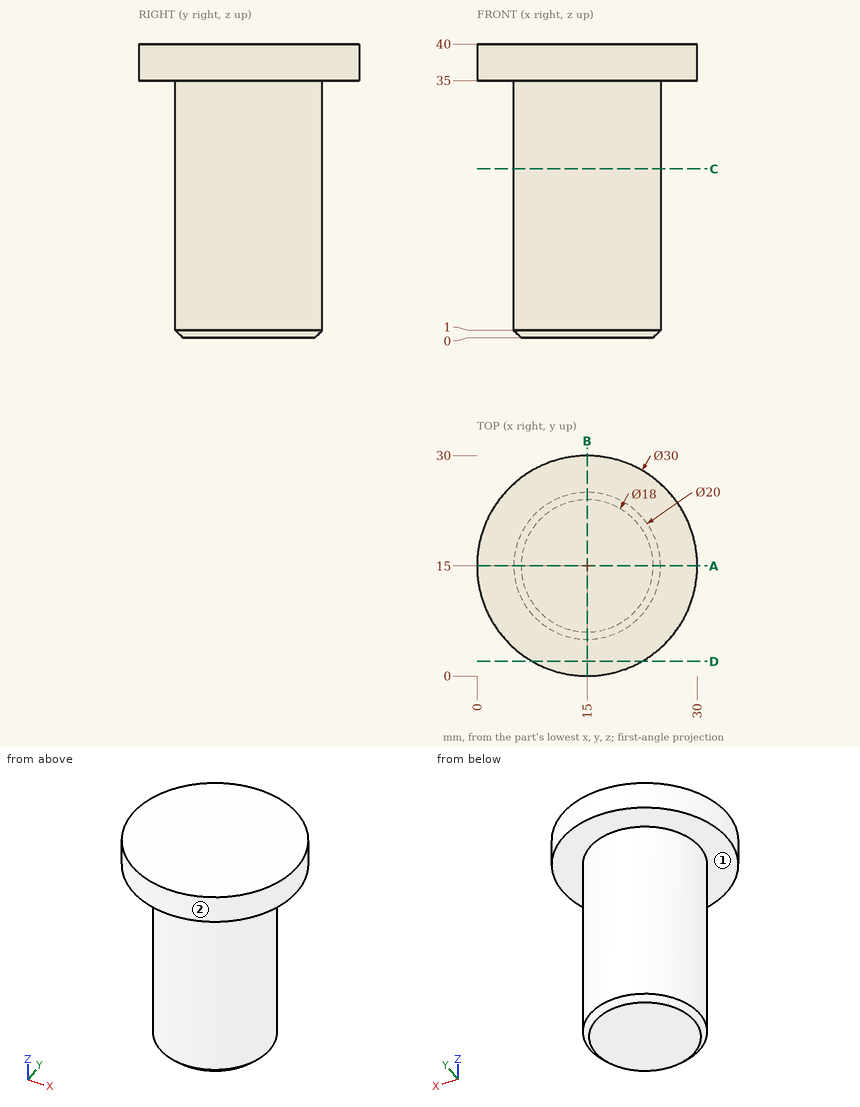
Design review of the part shown in the three views and the two pictorial views. Dimensions are in mm from the part's minimum x, y and z. A direction names the side the tool comes from. Coordinates: 2 decimals unless noted, no trailing zeros. Loops run counter-clockwise (first coordinate to the right, second up) from the corner with the lowest first, then second, coordinate; pieces in that order, holes last. Notation, with made-up numbers: (22.25, 83) - (59.25, 83) arc R10 ccw to (59.25, 88) - close; hole circle Ø11 at (82, 39.5). An arc over 180 degrees is marked (long way). Use a Markdown table: item, result. Add a question column.
Item 1: Tool access review of the marked faces 1 and 2: name each direction out of +Z, -Z, +X, -X, +Y, -Y from which nothing blocks a thin tool from reaching the whole face with its end or side.
Item 2: Insertion check: pin 1 Ø4 at (y, z) = (13, 4.5) entering from -X; pin 2 Ø5 at (y, z) = (17.5, 8.5) entering from +X; pin 3 Ø1 at (y, z) = (5.5, 30) entering from -X; pin 4 Ø1.5 at (x, y) = (11.5, 11.5) entering from -Z. Each pin has a flat end and moves straight along its axis. Give the tip position at first contact, or say it passes through.
Item 3: We need section A-A (y = 15). Give the boundary of the cut face in (x, z), and give its area (3 significant figures).
Item 4: For line 1 (Z direction, x = 16.25, y = 5); line 2 (Y direction, x = 15.25, z = 7.5); line 3 (Y direction, x = 13.75, z = 8), list the stretches that pass through material, from the lowest coordinate up.
Item 5: We need section D-D (y = 2). Give the boundary of the cut face in (x, z).
Item 6: We need section C-C (z = 23). Give the boundary of the cut face in (x, y), and give its area (3 significant figures).
Results list:
| question | item | result |
|---|---|---|
| 1 | face 1 | -Z |
| 1 | face 2 | +Z, -Z |
| 2 | pin 1 | stops at x = 5 |
| 2 | pin 2 | stops at x = 25 |
| 2 | pin 3 | stops at x = 10.64 |
| 2 | pin 4 | stops at z = 0 |
| 3 | outline | (0, 35) - (5, 35) - (5, 1) - (6, 0) - (24, 0) - (25, 1) - (25, 35) - (30, 35) - (30, 40) - (0, 40) - close |
| 3 | area | 849 mm^2 |
| 4 | line 1 | z = 35 to 40 |
| 4 | line 2 | y = 5 to 25 |
| 4 | line 3 | y = 5.08 to 24.92 |
| 5 | outline | (7.52, 35) - (22.48, 35) - (22.48, 40) - (7.52, 40) - close |
| 6 | outline | circle Ø20 at (15, 15) |
| 6 | area | 314 mm^2 |
